```python
from build123d import *

# Parameters (mm, degrees)
SKETCH_2_R             = 7.5
EXTRUDE_1_DEPTH        = 320
SKETCH_3_W             = 300
SKETCH_3_H             = 140
CUT_EXTRUDE_1_DEPTH    = 351.998575496
SKETCH_4_W             = 20
SKETCH_4_H             = 80
EXTRUDE_2_DEPTH        = 20
SKETCH_5_W             = 10
SKETCH_5_H             = 10
CUT_EXTRUDE_1480_DEPTH = 30
SKETCH_7_W             = 40
SKETCH_7_H             = 15
EXTRUDE_1842_DEPTH     = 20


with BuildPart() as part:
    # 草圖2 → 填料-伸長1 (new body)
    with BuildSketch(Plane(origin=(0, 0, 0), x_dir=(0, 0, -1), z_dir=(1, 0, 0))):
        with BuildLine():
            Line((-40, 0), (-40, -120))
            Line((-40, -120), (40, -120))
            Line((40, -120), (40, 0))
            ThreePointArc((40, 0), (0, 40), (-40, 0))
        make_face()
        Circle(SKETCH_2_R, mode=Mode.SUBTRACT)
    extrude(amount=EXTRUDE_1_DEPTH)

    # 草圖3 → 除料-伸長1 (cut, through all)
    with BuildSketch(Plane(origin=(0, 0, -40), x_dir=(-1, 0, 0), z_dir=(0, 0, -1))):
        with Locations((-160, -30)):
            Rectangle(SKETCH_3_W, SKETCH_3_H)
    extrude(amount=-CUT_EXTRUDE_1_DEPTH, mode=Mode.SUBTRACT)

    # 草圖4 → 填料-伸長2 (add)
    with BuildSketch(Plane.XZ.offset(120)):
        with Locations((10, 0)):
            Rectangle(SKETCH_4_W, SKETCH_4_H)
        with Locations((310, 0)):
            Rectangle(SKETCH_4_W, SKETCH_4_H)
    extrude(amount=EXTRUDE_2_DEPTH)

    # 草圖5 → Cut-Extrude 1480 (cut)
    with BuildSketch(Plane.XZ.offset(140)):
        with Locations((10, 0)):
            Rectangle(SKETCH_5_W, SKETCH_5_H)
        with Locations((310, 0)):
            Rectangle(SKETCH_5_W, SKETCH_5_H)
    extrude(amount=-CUT_EXTRUDE_1480_DEPTH, mode=Mode.SUBTRACT)

    # 草圖7 → Extrude 1842 (add)
    with BuildSketch(Plane(origin=(0, -100, 0), x_dir=(1, 0, 0), z_dir=(0, 1, 0))):
        with Locations((30, 32.5)):
            Rectangle(SKETCH_7_W, SKETCH_7_H)
        with Locations((30, -32.5)):
            Rectangle(SKETCH_7_W, SKETCH_7_H)
        with Locations((290, -32.5)):
            Rectangle(SKETCH_7_W, SKETCH_7_H)
        with Locations((290, 32.5)):
            Rectangle(SKETCH_7_W, SKETCH_7_H)
    extrude(amount=EXTRUDE_1842_DEPTH)


solid = part.part
```
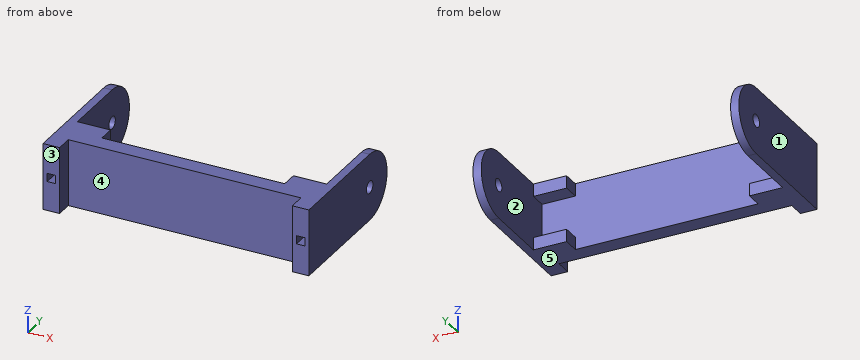
Check sheet for the modelled part. Datum: model origin and axes. Units: mm. Face numbers are marked on the shaded views. A direction names the side the tool comes from. Give positions to 0.01 mm unless a question says otherwise; leave off trailing zeros. Write each loop counter-clockwise with the first axis right and the second up, starting at its lowest first coordinate (ties: lowest second). Pieces come first, ordered by that corner, then holes.
Item 1: Cross-section at D-D (x = 38.5). Enter the section's corners in (y, z), and give its area (3 significant figures).
Item 2: Access from +Z, -Z, +X, -X, +Y, -Y to the whole of each face (thin tool, end or side, straight path). Record for the marked faces 4 and 5.
Item 3: Draft check along X on the marked faces 1, 2 and 3. Enter one of: released by +X, released by -X, zero draft, split by the parting line, or undercut.
Item 4: Cross-section at A-A (y = -124). Enter the section's corners in (x, z), and give its area (3 significant figures).
Item 5: Gauge pin test, flat ends, axial feed: pin 1 (24 mm diameter, centred on x = 205.5, z = -12, fed in from +Y); pin 2 (16.5 mm diameter, centred on x = 32, z = 34, fed in from +Y); pin 3 (10 mm diameter, centred on y = 12, z = -11, fed in from -X); pin 4 (1 mm diameter, centred on x = 186, z = -6.5, fed in from -Y). Record the tip position at first contact, or that the pin passes through.
Item 6: Cross-section at B-B (z = 0). Enter the section's corners in (x, y), and give its area (3 significant figures).
Item 7: Scan lines: L1, parallel to X at y = -129, z = -2.5; L2, parallel to X at y = -63, z = -6.5; L3, parallel to Y at x = 6.5, z = 0. Record each from-to range of solid material in increasing order.
Item 8: Cross-section at C-C (y = -75). Enter the section's corners in (x, z).
Report:
1. outline: (-120, -40) - (-80, -40) - (-80, -25) - (-100, -25) - (-100, 25) - (-80, 25) - (-80, 40) - (-120, 40) - close
1. area: 2,200 mm2
2. face 4: +Z, -Z, -Y
2. face 5: -Z, +X, -X, +Y, -Y
3. face 1: released by -X
3. face 2: undercut
3. face 3: zero draft
4. outline: (0, -40) - (20, -40) - (20, 40) - (0, 40) - close; (300, -40) - (320, -40) - (320, 40) - (300, 40) - close; hole (5, -5) - (15, -5) - (15, 5) - (5, 5) - close; hole (305, -5) - (315, -5) - (315, 5) - (305, 5) - close
4. area: 3,000 mm2
5. pin 1: stops at y = -100
5. pin 2: stops at y = -80
5. pin 3: stops at x = 0
5. pin 4: stops at y = -120
6. outline: (0, -140) - (5, -140) - (5, -110) - (15, -110) - (15, -140) - (20, -140) - (20, -120) - (300, -120) - (300, -140) - (305, -140) - (305, -110) - (315, -110) - (315, -140) - (320, -140) - (320, -7.5) - (310, -7.5) - (310, -100) - (10, -100) - (10, -7.5) - (0, -7.5) - close; (0, 7.5) - (10, 7.5) - (10, 40) - (0, 40) - close; (310, 7.5) - (320, 7.5) - (320, 40) - (310, 40) - close
6. area: 9,100 mm2
7. L1: x = 0 to 5, 15 to 20, 300 to 305, 315 to 320
7. L2: x = 0 to 10, 310 to 320
7. L3: y = -110 to -7.5, 7.5 to 40
8. outline: (0, -40) - (10, -40) - (10, 40) - (0, 40) - close; (310, -40) - (320, -40) - (320, 40) - (310, 40) - close
